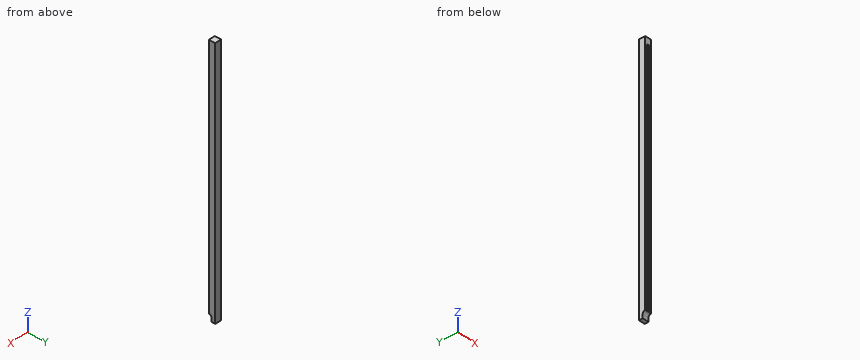
from build123d import *

# Parameters (mm, degrees)
F0_W     = 50
F0_H     = 50
F1_DEPTH = 2000
F2_W     = 20
F2_H     = 1900
F3_DEPTH = 15
F5_DEPTH = 50.001


with BuildPart() as f1:
    # F0 (on Top) → F1 (new body)
    with BuildSketch(Plane.XY):
        with Locations((25, 25)):
            Rectangle(F0_W, F0_H)
    extrude(amount=F1_DEPTH)

    # F2 (on Front) → F3 (cut)
    with BuildSketch(Plane.XZ):
        with Locations((25, 1000)):
            Rectangle(F2_W, F2_H)
    extrude(amount=-F3_DEPTH, mode=Mode.SUBTRACT)

    # F4 (on Right) → F5 (cut, through all)
    with BuildSketch(Plane.YZ):
        with BuildLine():
            Line((0, 50), (0, 0))
            Line((0, 0), (20, 0))
            Line((20, 0), (20, 30))
            ThreePointArc((20, 30), (14.142136, 44.142136), (0, 50))
        make_face()
    extrude(amount=F5_DEPTH, mode=Mode.SUBTRACT)


solid = f1.part
Input: part model. Units: mm. Frame: model coordinates. Round coordinates to 2 decimals unless told otherwise and drop trailing zeros. Loops run counter-clockwise (first coordinate to the right, second up) from the corner with the lowest first, then second, coordinate; pieces in that order, holes last. Notation, with made-up numbers: (40, 41.5) -> (70, 41.5) arc R32 ccw to (70, 79.5) -> close; hole circle Ø9 at (47.5, -5). An arc over 180 degrees is marked (long way). Answer as a JSON object with one key per item and string values. Group by question number.
1) Ray query, L1, parallel to X at y = 7, z = 505; L2, parallel to Y at x = 20.5, z = 650.5; L3, parallel to Z at x = 17, y = 7 (3 decimals). Return the intervals inside material, ascending.
2) Section query A-A on z = 335.5. Output: boundary loops of the cut face in (x, y), plus the area to 3 significant figures.
3) Pin query (flat end, axial travel): pin 1 (12 mm diameter, centred on x = 26, y = 4.5, fed in from -Z); pin 2 (2 mm diameter, centred on x = 17.5, y = 7, fed in from -Z). Return the tip coordinate at first contact, or that it passes through.
Reply:
{
 "1": {"L1": "x = 0 to 15, 35 to 50", "L2": "y = 15 to 50", "L3": "z = 48.735 to 50, 1950 to 2000"},
 "2": {"outline": "(0, 0) -> (15, 0) -> (15, 15) -> (35, 15) -> (35, 0) -> (50, 0) -> (50, 50) -> (0, 50) -> close", "area": "2,200 mm2"},
 "3": {"pin 1": "stops at z = 47.02", "pin 2": "stops at z = 48.33"}
}
